from build123d import *

# Parameters (mm, degrees)
F0_W     = 26.1790351942
F0_H     = 15.7074220479
F0_H_2   = 36.0050015152
F0_W_2   = 25.6373991724
F1_DEPTH = 52.07
F2_R     = 1.8396307345


with BuildPart() as f1:
    # F0 (on Front) → F1 (new body)
    with BuildSketch(Plane.XZ):
        with Locations((27.227526065, 43.8587125391)):
            Rectangle(F0_W, F0_H)
        with Locations((27.227526065, 18.0025007576)):
            Rectangle(F0_W, F0_H_2)
        Polygon((-28.8317184895, 36.0050015152), (-28.8317184895, 0), (14.1380084679, 0), (14.1380084679, 36.0050015152), (-3.1943193171, 36.0050015152), align=None)
        with Locations((-16.0130189033, 43.8587125391)):
            Rectangle(F0_W_2, F0_H)
        Polygon((-75.5928903818, 51.712423563), (-75.5928903818, 0), (-28.8317184895, 0), (-28.8317184895, 36.0050015152), (-28.8317184895, 51.712423563), align=None)
    extrude(amount=F1_DEPTH)

    # F2
    f2_edges = [f1.edges().sort_by_distance(p)[0] for p in [
        (14.138008, 0, 43.858713),
        (5.471845, 0, 36.005002),
        (-3.194319, 0, 43.858713),
        (-39.393605, 0, 51.712424),
        (-75.59289, 0, 25.856212),
        (-17.637923, 0, 0),
        (40.317044, 0, 25.856212),
        (27.227526, 0, 51.712424),
        (14.138008, -52.07, 43.858713),
        (5.471845, -52.07, 36.005002),
        (-3.194319, -52.07, 43.858713),
        (-39.393605, -52.07, 51.712424),
        (-75.59289, -52.07, 25.856212),
        (-17.637923, -52.07, 0),
        (40.317044, -52.07, 25.856212),
        (27.227526, -52.07, 51.712424),
        (40.317044, -26.035, 0),
        (40.317044, -26.035, 51.712424),
        (-75.59289, -26.035, 51.712424),
        (-75.59289, -26.035, 0),
    ]]
    fillet(f2_edges, radius=F2_R)


solid = f1.part
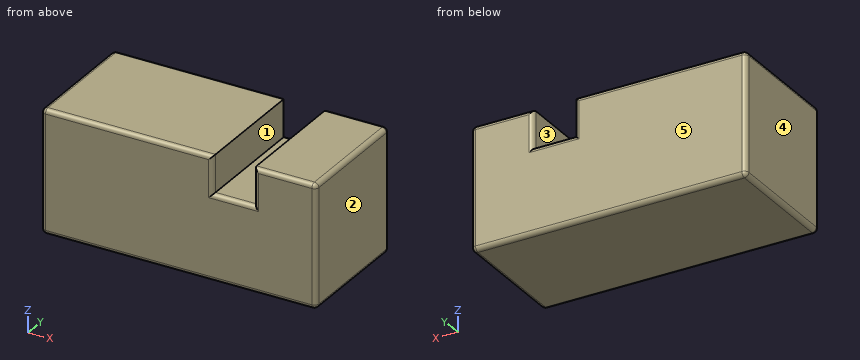
Check sheet for the modelled part. Datum: model origin and axes. Units: mm. Face numbers are marked on the shaded views. A direction names the side the tool comes from. Give positions to 0.01 mm unless a question says otherwise; leave off trailing zeros. Loops run counter-clockwise (first coordinate to the right, second up) from the corner with the lowest first, then second, coordinate; pieces in that order, holes last. Notation, with made-up numbers: M 57,3.5 L 90,3.5 A28 cw 90,31.5 Z; hole C -40,43 d10. An arc over 180 degrees is marked long. Return JSON: item names as keys, results as strings. Group by question number.
1. Cross-section at B-B on y = -32.5. Record the boundary of the cut face in (x, z) (3 decimals).
2. Tool access check on the marked faces 1 and 2. Record the directions out of +Z, -Z, +X, -X, +Y, -Y that give a thin tool (end or side, any length) a straight path to the whole face; none if there is none.
3. Mould release check, pull along X, two halves, no side actions. Record for the marked faces 3, 4 and 5: released by +X, released by -X, zero draft, split by the parting line, or undercut.
4. Cross-section at A-A on z = 38. Record the boundary of the cut face in (x, y), plus the area to 3 significant figures.
5. Thickness scan on L1, parallel to X at y = -5.5, z = 43.5; L2, parallel to Z at x = -2.5, y = -34.5 (3 decimals). Record the ranges inside material, lowest first.
6. Go/stop test with a flat-tipped pin: pin 1 (5 mm diameter, centred on x = 4.5, y = -23, fed in from +Z) (3 decimals). Record where the tip stops, or that it passes through.
Return value:
{
 "1": {"outline": "M -75.593,1.84 A1.84 ccw -73.753,0 L 38.477,0 A1.84 ccw 40.317,1.84 L 40.317,49.873 A1.84 ccw 38.477,51.712 L 14.138,51.712 L 14.138,36.005 L -3.194,36.005 L -3.194,51.712 L -73.753,51.712 A1.84 ccw -75.593,49.873 Z"},
 "2": {"face 1": "+Z, +Y, -Y", "face 2": "+Z, -Z, +X, +Y, -Y"},
 "3": {"face 3": "undercut", "face 4": "released by -X", "face 5": "zero draft"},
 "4": {"outline": "M -75.59,-50.23 A1.84 ccw -73.75,-52.07 L -5.03,-52.07 A1.84 ccw -3.19,-50.23 L -3.19,-1.84 A1.84 ccw -5.03,0 L -73.75,0 A1.84 ccw -75.59,-1.84 Z; M 14.14,-50.23 A1.84 ccw 15.98,-52.07 L 38.48,-52.07 A1.84 ccw 40.32,-50.23 L 40.32,-1.84 A1.84 ccw 38.48,0 L 15.98,0 A1.84 ccw 14.14,-1.84 Z", "area": "5,130 mm^2"},
 "5": {"L1": "-75.59 to -3.19, 14.14 to 40.32", "L2": "0 to 36.005"},
 "6": {"pin 1": "z = 36.005"}
}
